Autodesk Inventor part; units mm, degrees
ref_plane "Work Plane1" through (0, 16, 0) normal (0, 1, 0) x (-1, 0, 0)
ref_plane "Work Plane2" through (0, 14.5, 0) normal (0, 1, 0) x (-1, 0, 0)
ref_plane "Work Plane3" through (0, 11.5, 0) normal (0, 1, 0) x (1, 0, 0)
ref_plane "Work Plane1" through (0, 16, 0) normal (0, 1, 0) x (-1, 0, 0)
sketch "Sketch1" plane through (0, 16, 0) normal (0, 1, 0) x (-1, 0, 0)
  circle A0 centre (0, 0) radius 9
extrude "Extrusion3" add sketch "Sketch1" against normal blind 16
ref_plane "Work Plane2" through (0, 14.5, 0) normal (0, 1, 0) x (-1, 0, 0)
sketch "Sketch2" plane through (0, 14.5, 0) normal (0, 1, 0) x (-1, 0, 0)
  arc A0 (4.4703, 2.987) -> (3.8017, 3.8017) centre (0, 0) ccw
  line L0 (2.987, -4.4703) -> (3.5426, -5.3018)
  arc A1 (-5.8911, -2.4402) -> (-5.3018, -3.5426) centre (0, 0) ccw
  line L1 (-2.4402, 5.8911) -> (-2.0575, 4.9672)
  line L2 (2.987, 4.4703) -> (3.5426, 5.3018)
  arc A2 (4.5088, -4.5088) -> (5.3018, -3.5426) centre (0, 0) ccw
  line L3 (-4.5088, -4.5088) -> (-3.8017, -3.8017)
  arc A3 (-2.987, 4.4703) -> (-3.8017, 3.8017) centre (0, 0) ccw
  arc A4 (2.4402, 5.8911) -> (1.244, 6.2539) centre (0, 0) ccw
  line L4 (5.8911, -2.4402) -> (4.9672, -2.0575)
  arc A5 (-2.987, -4.4703) -> (-2.0575, -4.9672) centre (0, 0) ccw
  line L5 (-4.4703, 2.987) -> (-5.3018, 3.5426)
  line L6 (0, 6.3764) -> (0, 5.3764)
  arc A6 (5.2731, -1.0489) -> (5.3764, 0) centre (0, 0) ccw
  line L7 (-1.0489, -5.2731) -> (-1.244, -6.2539)
  arc A7 (-5.8911, 2.4402) -> (-6.2539, 1.244) centre (0, 0) ccw
  line L8 (5.2731, 1.0489) -> (6.2539, 1.244)
  arc A8 (0, -6.3764) -> (1.244, -6.2539) centre (0, 0) ccw
  line L9 (-6.3764, 0) -> (-5.3764, 0)
  arc A9 (5.8911, 2.4402) -> (5.3018, 3.5426) centre (0, 0) ccw
  line L10 (2.4402, -5.8911) -> (2.0575, -4.9672)
  arc A10 (-5.2731, -1.0489) -> (-4.9672, -2.0575) centre (0, 0) ccw
  line L11 (-1.0489, 5.2731) -> (-1.244, 6.2539)
  line L12 (4.5088, 4.5088) -> (3.8017, 3.8017)
  arc A11 (2.987, -4.4703) -> (3.8017, -3.8017) centre (0, 0) ccw
  line L13 (-4.4703, -2.987) -> (-5.3018, -3.5426)
  arc A12 (-2.4402, 5.8911) -> (-3.5426, 5.3018) centre (0, 0) ccw
  arc A13 (2.987, 4.4703) -> (2.0575, 4.9672) centre (0, 0) ccw
  line L14 (4.4703, -2.987) -> (5.3018, -3.5426)
  arc A14 (-4.5088, -4.5088) -> (-3.5426, -5.3018) centre (0, 0) ccw
  line L15 (-4.5088, 4.5088) -> (-3.8017, 3.8017)
  line L16 (1.0489, 5.2731) -> (1.244, 6.2539)
  arc A15 (5.8911, -2.4402) -> (6.2539, -1.244) centre (0, 0) ccw
  line L17 (-2.4402, -5.8911) -> (-2.0575, -4.9672)
  arc A16 (-4.4703, 2.987) -> (-4.9672, 2.0575) centre (0, 0) ccw
  arc A17 (0, 6.3764) -> (-1.244, 6.2539) centre (0, 0) ccw
  line L18 (6.3764, 0) -> (5.3764, 0)
  arc A18 (-1.0489, -5.2731) -> (0, -5.3764) centre (0, 0) ccw
  line L19 (-5.2731, 1.0489) -> (-6.2539, 1.244)
  arc A19 (5.2731, 1.0489) -> (4.9672, 2.0575) centre (0, 0) ccw
  line L20 (1.0489, -5.2731) -> (1.244, -6.2539)
  arc A20 (-6.3764, 0) -> (-6.2539, -1.244) centre (0, 0) ccw
  line L21 (4.4703, 2.987) -> (5.3018, 3.5426)
  arc A21 (2.4402, -5.8911) -> (3.5426, -5.3018) centre (0, 0) ccw
  line L22 (-5.8911, -2.4402) -> (-4.9672, -2.0575)
  arc A22 (-1.0489, 5.2731) -> (-2.0575, 4.9672) centre (0, 0) ccw
  arc A23 (4.5088, 4.5088) -> (3.5426, 5.3018) centre (0, 0) ccw
  line L23 (4.5088, -4.5088) -> (3.8017, -3.8017)
  arc A24 (-4.4703, -2.987) -> (-3.8017, -3.8017) centre (0, 0) ccw
  line L24 (-2.987, 4.4703) -> (-3.5426, 5.3018)
  line L25 (2.4402, 5.8911) -> (2.0575, 4.9672)
  arc A25 (4.4703, -2.987) -> (4.9672, -2.0575) centre (0, 0) ccw
  line L26 (-2.987, -4.4703) -> (-3.5426, -5.3018)
  arc A26 (-4.5088, 4.5088) -> (-5.3018, 3.5426) centre (0, 0) ccw
  arc A27 (1.0489, 5.2731) -> (0, 5.3764) centre (0, 0) ccw
  line L27 (5.2731, -1.0489) -> (6.2539, -1.244)
  arc A28 (-2.4402, -5.8911) -> (-1.244, -6.2539) centre (0, 0) ccw
  line L28 (-5.8911, 2.4402) -> (-4.9672, 2.0575)
  circle A29 centre (0, 0) radius 9
  arc A30 (6.3764, 0) -> (6.2539, 1.244) centre (0, 0) ccw
  line L29 (0, -6.3764) -> (0, -5.3764)
  arc A31 (-5.2731, 1.0489) -> (-5.3764, 0) centre (0, 0) ccw
  line L30 (5.8911, 2.4402) -> (4.9672, 2.0575)
  arc A32 (1.0489, -5.2731) -> (2.0575, -4.9672) centre (0, 0) ccw
  line L31 (-5.2731, -1.0489) -> (-6.2539, -1.244)
extrude "Extrusion2" cut sketch "Sketch2" against normal blind 6
sketch "Sketch3" plane through (0, 0, 0) normal (0, 1, 0) x (-1, 0, 0)
  circle A0 centre (0, 0) radius 2.5
extrude "Extrusion1" cut sketch "Sketch3" along normal blind 16
ref_plane "Work Plane3" through (0, 11.5, 0) normal (0, 1, 0) x (1, 0, 0)
properties part number "T2.5 16T Pulley" material "Aluminum 6061"
Build history of the part. All positions in model axes, mm. A direction names the side the tool comes from. Round coordinates to 2 decimals unless told otherwise and drop trailing zeros. Write each loop counter-clockwise with the first axis right and the second up, starting at its lowest first coordinate (ties: lowest second). Pieces come first, ordered by that corner, then holes. Notation, with made-up numbers: M 23,48 L 31,48 A22 ccw 31,81 Z; hole C 36,59 d7. An arc over 180 degrees is marked long. Answer as a JSON object with one key per item and string values. Group by question number.
(1) Mould opens along Y. For faces 1 (the cylindrical face through (1.172, 15.26, 8.923)), 2 (the cylindrical face through (2.998, 11.542, 5.628)), 3 (the cylindrical face through (4.923, 11.542, 4.052)) say: pulls with the +Y half, pulls with the -Y half, needs draft (parallel to the pull), parting line crosses it, or undercut.
(2) Cut at D-D (z = 3.25). Give the cut face in (x, y).
(3) Cut at B-B (x = -1.5). Give the cut face in (y, z).
(4) Drill centre lines: L1, parallel to Z at x = 0, y = 7.5; L2, parallel to Y at x = 7.75, z = 2; L3, parallel to Z at x = -1, y = 8.25. Where is each one in solid material? Low to high.
(5) Cut at C-C (y = 3.25). Give the cut face in (x, z), and give its area (3 significant figures).
(6) Cut at A-A (z = 7). Give the cut face in (x, y).
(7) Which spindle directions (+Z, -Z, +X, -X, +Y, -Y) get a long thin tool onto all of the face, cutting with end or side? Do faces 4 (the cylindrical face through (1.86, 11.54, -6.1)), 5 (the cylindrical face through (-4.052, 11.542, 4.923)), 6 (the cylindrical face through (1.55, 11.54, 5.15)), 7 (the cylindrical face through (0.53, 11.54, -5.35)). Say none if no direction does.
(8) Flat gauge pins, fed straight in: pin 1 (0.5 mm diameter, centred on x = -6, y = 11.5, fed in from -Z); pin 2 (6 mm diameter, centred on y = 13, z = -6.5, fed in from -X); pin 3 (1.1 mm diameter, centred on x = 6, y = 11.5, fed in from +Z); pin 4 (6 mm diameter, centred on x = -0.5, z = 0.5, fed in from +Y). Where does each tip first touch, or does it go through?
Responses:
{
 "1": {"face 1": "needs draft", "face 2": "undercut", "face 3": "undercut"},
 "2": {"outline": "M -8.39,0 L 8.39,0 L 8.39,8.5 L 4.86,8.5 L 4.86,14.5 L 8.39,14.5 L 8.39,16 L -8.39,16 L -8.39,14.5 L -5.49,14.5 L -5.49,8.5 L -8.39,8.5 Z; hole M -4.86,8.5 L -4.28,8.5 L -4.28,14.5 L -4.86,14.5 Z"},
 "3": {"outline": "M 0,-8.87 L 8.5,-8.87 L 8.5,-5.16 L 14.5,-5.16 L 14.5,-8.87 L 16,-8.87 L 16,-2 L 0,-2 Z; M 0,2 L 16,2 L 16,8.87 L 14.5,8.87 L 14.5,6.2 L 8.5,6.2 L 8.5,8.87 L 0,8.87 Z"},
 "4": {"L1": "z = -9 to -2.5, 2.5 to 9", "L2": "y = 0 to 8.5, 14.5 to 16", "L3": "z = -8.94 to -2.29, 2.29 to 8.94"},
 "5": {"outline": "C 0,0 d18; hole C 0,0 d5", "area": "235 mm2"},
 "6": {"outline": "M -5.66,0 L 5.66,0 L 5.66,8.5 L -5.66,8.5 Z; M -5.66,14.5 L 5.66,14.5 L 5.66,16 L -5.66,16 Z"},
 "7": {"face 4": "-Z, +X", "face 5": "+Z, -X", "face 6": "none", "face 7": "-Z"},
 "8": {"pin 1": "stops at z = -2.44", "pin 2": "stops at x = -8.11", "pin 3": "stops at z = 2.44", "pin 4": "stops at y = 16"}
}
